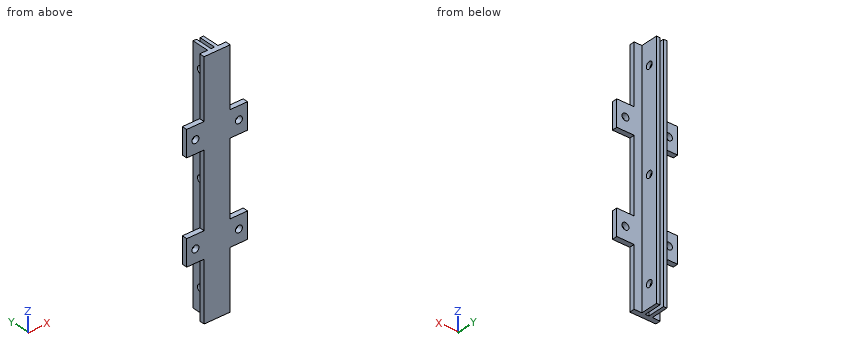
```python
from build123d import *

# Parameters (mm, degrees)
BOSS_EXTRUDE1_DEPTH = 5
BOSS_EXTRUDE2_DEPTH = 3
SKETCH3_W           = 2
SKETCH3_H           = 170
BOSS_EXTRUDE3_DEPTH = 10
SKETCH5_R           = 2
CUT_EXTRUDE1_DEPTH  = 10
SKETCH6_R           = 2
CUT_EXTRUDE3_DEPTH  = 5
SKETCH8_W           = 55
SKETCH8_H           = 14.626241735
CUT_EXTRUDE4_DEPTH  = 20
SKETCH9_W           = 140.74751653
SKETCH9_H           = 5
CUT_EXTRUDE5_DEPTH  = 300


with BuildPart() as part:
    # Sketch1 → Boss-Extrude1 (new body)
    with BuildSketch(Plane(origin=(0, 0, 0), x_dir=(1, 0, 0), z_dir=(0, 1, 0))):
        with BuildLine():
            Line((-27.5, 42.873758265), (-27.5, 13.75))
            ThreePointArc((-27.5, 13.75), (-13.75, 0), (-27.5, -13.75))
            Line((-27.5, -13.75), (-27.5, -42.873758265))
            ThreePointArc((-27.5, -42.873758265), (-13.75, -56.623758265), (-27.5, -70.373758265))
            Line((-27.5, -70.373758265), (-27.5, -85))
            Line((-27.5, -85), (27.5, -85))
            Line((27.5, -85), (27.5, -70.373758265))
            ThreePointArc((27.5, -70.373758265), (13.75, -56.623758265), (27.5, -42.873758265))
            Line((27.5, -42.873758265), (27.5, -13.75))
            ThreePointArc((27.5, -13.75), (13.75, 0), (27.5, 13.75))
            Line((27.5, 13.75), (27.5, 42.873758265))
            ThreePointArc((27.5, 42.873758265), (13.75, 56.623758265), (27.5, 70.373758265))
            Line((27.5, 70.373758265), (27.5, 85))
            Line((27.5, 85), (-27.5, 85))
            Line((-27.5, 85), (-27.5, 70.373758265))
            ThreePointArc((-27.5, 70.373758265), (-13.75, 56.623758265), (-27.5, 42.873758265))
        make_face()
    extrude(amount=BOSS_EXTRUDE1_DEPTH)

    # Sketch2 → Boss-Extrude2 (add)
    with BuildSketch(Plane(origin=(0, 5, 0), x_dir=(1, 0, 0), z_dir=(0, 1, 0))):
        Polygon((-7.5, 85), (7.5, 85), (7.5, 36.25), (17.5, 36.25), (17.5, 21.25), (7.5, 21.25), (7.5, -21.25), (17.5, -21.25), (17.5, -36.25), (7.5, -36.25), (7.5, -85), (-7.5, -85), (-7.5, -36.25), (-17.5, -36.25), (-17.5, -21.25), (-7.5, -21.25), (-7.5, 21.25), (-17.5, 21.25), (-17.5, 36.25), (-7.5, 36.25), align=None)
    extrude(amount=BOSS_EXTRUDE2_DEPTH)

    # Sketch3 → Boss-Extrude3 (add)
    with BuildSketch(Plane(origin=(0, 8, 0), x_dir=(1, 0, 0), z_dir=(0, 1, 0))):
        with Locations((-2, 0)):
            Rectangle(SKETCH3_W, SKETCH3_H)
        with Locations((2, 0)):
            Rectangle(SKETCH3_W, SKETCH3_H)
    extrude(amount=BOSS_EXTRUDE3_DEPTH)

    # Sketch5 → Cut-Extrude1 (cut)
    with BuildSketch(Plane.ZY.offset(3)):
        with Locations((0, 13)):
            Circle(SKETCH5_R)
        with Locations((-57.5, 13)):
            Circle(SKETCH5_R)
        with Locations((57.5, 13)):
            Circle(SKETCH5_R)
    extrude(amount=-CUT_EXTRUDE1_DEPTH, mode=Mode.SUBTRACT)

    # Sketch6 → Cut-Extrude3 (cut)
    with BuildSketch(Plane(origin=(0, 8, 0), x_dir=(1, 0, 0), z_dir=(0, 1, 0))):
        with Locations(Location((-12.5, 28.75, 0), (0, 0, 270))):
            Circle(SKETCH6_R)
        with Locations(Location((12.5, 28.75, 0), (0, 0, 90))):
            Circle(SKETCH6_R)
        with Locations(Location((12.5, -28.75, 0), (0, 0, 270))):
            Circle(SKETCH6_R)
        with Locations(Location((-12.5, -28.75, 0), (0, 0, 90))):
            Circle(SKETCH6_R)
    extrude(amount=-CUT_EXTRUDE3_DEPTH, mode=Mode.SUBTRACT)

    # Sketch8 → Cut-Extrude4 (cut)
    with BuildSketch(Plane(origin=(0, 18, 0), x_dir=(1, 0, 0), z_dir=(0, 1, 0))):
        with Locations((0, 77.686879132)):
            Rectangle(SKETCH8_W, SKETCH8_H)
        with Locations((0, -77.686879132)):
            Rectangle(SKETCH8_W, SKETCH8_H)
    extrude(amount=-CUT_EXTRUDE4_DEPTH, mode=Mode.SUBTRACT)

    # Sketch9 → Cut-Extrude5 (cut)
    with BuildSketch(Plane.ZY.offset(27.5)):
        with Locations((0, 2.5)):
            Rectangle(SKETCH9_W, SKETCH9_H)
    extrude(amount=-CUT_EXTRUDE5_DEPTH, mode=Mode.SUBTRACT)


solid = part.part
```
Geometry check sheet. Reference: the model listing, model coordinates, mm. Coordinates: 2 decimals unless noted, no trailing zeros. Order: outer loops, then holes, each group sorted by start corner. A loop starts at its lowest first (then second) coordinate and runs counter-clockwise, first axis right, second up. Notation, with made-up numbers: (-5.5, -11) - (28.5, -11) arc R37 ccw to (28.5, 26) - close; hole circle Ø3 at (-8, 25.25). An arc over 180 degrees is marked (long way). Use one line per item in the form item = value.
1. Section check B-B (y = 13). State how many separate pieces and enclosed holes the cut face has, then the cut area to 3 significant figures.
Here are the results:
separate_pieces = 8
enclosed_holes = 0
area = 515 mm²
2. Gauge pin test, flat ends, axial feed: pin 1 (3.5 mm diameter, centred on x = 13.5, y = 6, fed in from -Z); pin 2 (1.5 mm diameter, centred on y = 6, z = 5, fed in from +X); pin 3 (4.5 mm diameter, centred on y = 13, z = 57.5, fed in from +X). Record the tip position at first contact, or that the pin passes through.
Here are the results:
pin_1 = -36.25
pin_2 = 7.5
pin_3 = 3
3. Scan lines: line 1 (X direction, y = 6.35, z = -28.75); line 2 (Y direction, x = -2, z = 0); line 3 (X direction, y = 8.5, z = -29). Record each from-to range of solid material in increasing order.
Here are the results:
line_1 = -17.5 to -14.5, -10.5 to 10.5, 14.5 to 17.5
line_2 = 5 to 11, 15 to 18
line_3 = -3 to -1, 1 to 3
4. Section check C-C (x = -12.5). Record the boundary of the cut face in (y, z).
Here are the results:
outline = (5, -36.25) - (8, -36.25) - (8, -30.75) - (5, -30.75) - close; (5, -26.75) - (8, -26.75) - (8, -21.25) - (5, -21.25) - close; (5, 21.25) - (8, 21.25) - (8, 26.75) - (5, 26.75) - close; (5, 30.75) - (8, 30.75) - (8, 36.25) - (5, 36.25) - close
5. Section check D-D (z = 43). Record the boundary of the cut face in (x, y), then the cut area to 3 significant figures.
Here are the results:
outline = (-7.5, 5) - (7.5, 5) - (7.5, 8) - (3, 8) - (3, 18) - (1, 18) - (1, 8) - (-1, 8) - (-1, 18) - (-3, 18) - (-3, 8) - (-7.5, 8) - close
area = 85.0 mm²
6. Section check A-A (z = -57.5). Record the boundary of the cut face in (x, y).
Here are the results:
outline = (-7.5, 5) - (7.5, 5) - (7.5, 8) - (3, 8) - (3, 11) - (1, 11) - (1, 8) - (-1, 8) - (-1, 11) - (-3, 11) - (-3, 8) - (-7.5, 8) - close; (-3, 15) - (-1, 15) - (-1, 18) - (-3, 18) - close; (1, 15) - (3, 15) - (3, 18) - (1, 18) - close
